The listing builds one solid part. Answer for the finished solid, in the listing's coordinates (mm). A direction names the side the tool comes from. Coordinates: 2 decimals unless noted, no trailing zeros. Write each loop counter-clockwise with the first axis right and the second up, starting at its lowest first coordinate (ties: lowest second). Pieces come first, ordered by that corner, then holes.
from build123d import *

# Parameters (mm, degrees)
F0_R     = 5.5
F0_R_2   = 3.75
F0_R_3   = 4
F1_DEPTH = 2
F2_DEPTH = 12
F3_DEPTH = 1
F4_ANGLE = 90


with BuildPart() as f1:
    # F0 (on Front) → F1 (new body)
    with BuildSketch(Plane.XZ):
        with BuildLine():
            ThreePointArc((20.6234359139, 1.0467505913), (25, 4.5), (29.3765640861, 1.0467505913))
            ThreePointArc((29.3765640861, 1.0467505913), (29.8140239679, -0.117408547), (30.5252627854, -1.1375933304))
            Line((30.5252627854, -1.1375933304), (32.5105844978, -3.3404322227))
            ThreePointArc((32.5105844978, -3.3404322227), (34.1921257049, -4.5612374621), (36.2247347829, -4.9930320884))
            Line((36.2247347829, -4.9930320884), (50, -4.9930320884))
            ThreePointArc((50, -4.9930320884), (60.4567630389, 14.3557712193), (38.5413898737, 12.5019908319))
            ThreePointArc((38.5413898737, 12.5019908319), (36.6974671463, 10.3172947844), (33.9579458232, 9.5))
            Line((33.9579458232, 9.5), (-33.9579458232, 9.5))
            ThreePointArc((-33.9579458232, 9.5), (-36.6974671463, 10.3172947844), (-38.5413898737, 12.5019908319))
            ThreePointArc((-38.5413898737, 12.5019908319), (-60.4567630389, 14.3557712193), (-50, -4.9930320884))
            Line((-50, -4.9930320884), (-36.224734783, -4.9930320884))
            ThreePointArc((-36.224734783, -4.9930320884), (-34.1921257049, -4.5612374621), (-32.5105844978, -3.3404322227))
            Line((-32.5105844978, -3.3404322227), (-30.5252627854, -1.1375933304))
            ThreePointArc((-30.5252627854, -1.1375933304), (-29.8140239679, -0.117408547), (-29.3765640861, 1.0467505913))
            ThreePointArc((-29.3765640861, 1.0467505913), (-25, 4.5), (-20.6234359139, 1.0467505913))
            ThreePointArc((-20.6234359139, 1.0467505913), (-20.1859760321, -0.117408547), (-19.4747372146, -1.1375933304))
            Line((-19.4747372146, -1.1375933304), (-17.4894155022, -3.3404322227))
            ThreePointArc((-17.4894155022, -3.3404322227), (-15.8078742951, -4.5612374621), (-13.775265217, -4.9930320884))
            Line((-13.775265217, -4.9930320884), (13.775265217, -4.9930320884))
            ThreePointArc((13.775265217, -4.9930320884), (15.8078742951, -4.5612374621), (17.4894155022, -3.3404322227))
            Line((17.4894155022, -3.3404322227), (19.4747372146, -1.1375933304))
            ThreePointArc((19.4747372146, -1.1375933304), (20.1859760321, -0.117408547), (20.6234359139, 1.0467505913))
        make_face()
        with Locations((-50, 7.5069679116)):
            Circle(F0_R, mode=Mode.SUBTRACT)
        with Locations((50, 7.5069679116)):
            Circle(F0_R, mode=Mode.SUBTRACT)
        with Locations((-50, 7.5069679116)):
            Circle(F0_R)
        with Locations((-50, 7.5069679116)):
            Circle(F0_R_2, mode=Mode.SUBTRACT)
        with Locations((50, 7.5069679116)):
            Circle(F0_R)
        with Locations((50, 7.5069679116)):
            Circle(F0_R_3, mode=Mode.SUBTRACT)
        with Locations((-50, 7.5069679116)):
            Circle(F0_R_2)
    extrude(amount=F1_DEPTH)

    # F0 (on Front) → F2 (join)
    with BuildSketch(Plane.XZ):
        with Locations((-50, 7.5069679116)):
            Circle(F0_R_2)
    extrude(amount=-F2_DEPTH)

    # F0 (on Front) → F3 (join)
    with BuildSketch(Plane.XZ):
        with Locations((-50, 7.5069679116)):
            Circle(F0_R)
        with Locations((-50, 7.5069679116)):
            Circle(F0_R_2, mode=Mode.SUBTRACT)
        with Locations((50, 7.5069679116)):
            Circle(F0_R)
        with Locations((50, 7.5069679116)):
            Circle(F0_R_3, mode=Mode.SUBTRACT)
    extrude(amount=-F3_DEPTH)


with BuildPart() as f1_1:
    # F4: moved
    add(f1.part.rotate(Axis((0, 0, 9.5), (1, 0, 0)), F4_ANGLE))


solid = f1_1.part
1. Section A-A on x = 43 is taken. Give the vertices of the cut face in (y, z).
Results found:
outline: (-8.36, 7.5) - (14.49, 7.5) - (14.49, 9.5) - (-8.36, 9.5) - close
2. Find the intervals of material crossed by L1, parallel to Y at x = 50, z = 8.7; L2, parallel to Y at x = 50, z = 9.7; L3, parallel to Z at x = -6.5, y = 0.5, in increasing order.
Results found:
L1: y = -10.51 to -2.01, 5.99 to 14.49
L2: y = -3.51 to -2.01, 5.99 to 7.49
L3: z = 7.5 to 9.5
3. Section B-B on z = 16.25 is taken. Give the vertices of the cut face in (x, y).
Results found:
outline: circle Ø7.5 at (-50, 1.99)
4. A tool of negligible diameter and unlimited length cuts with its end or side. For faces 1 (the flat face through (-46, 3, 10.5)), 2 (the cylindrical face through (36.73, -0.84, 8.51)), 3 (the cylindrical face through (-34.219, 14.073, 8.514)), 4 (the cylindrical face through (-60.246, -5.167, 8.514)), from which of +Z, -Z, +X, -X, +Y, -Y can it reach the whole face along a straight path? Write none if from no direction.
Results found:
face 1: +Z
face 2: +Z, -Z, -Y
face 3: +Z, -Z, +Y
face 4: +Z, -Z
5. Flat-ended cylindrical pins translate along their axes: P1, Ø1.6, axis at x = 13, z = 8, coming from the -Y side; P2, Ø3, axis at x = 39, y = -0.5, coming from the +Z side; P3, Ø12, axis at x = 48.5, y = 1, coming from the +Z side. Find the tip coordinate at first contact, or state that the pin passes through.
Results found:
P1: stops at y = 0
P2: stops at z = 9.5
P3: stops at z = 10.5
6. For a pull along Y with two mould halves and no side action, classify faces 5 (the cylindrical face through (46, 2, 9)), 6 (the cylindrical face through (60.658, -4.538, 8.514)), 7 (the flat face through (18.47, 11.75, 8.51)) as pulls with the +Y half, pulls with the -Y half, needs draft (parallel to the pull), parting line crosses it, or undercut.
Results found:
face 5: undercut
face 6: parting line crosses it
face 7: pulls with the +Y half
